For this review, take the finished solid that the model builds, in its own axes (mm). Face numbers are marked on the shaded views. A direction names the side the tool comes from. Coordinates: 2 decimals unless noted, no trailing zeros. Write each loop counter-clockwise with the first axis right and the second up, starting at its lowest first coordinate (ties: lowest second). Pieces come first, ordered by that corner, then holes. Notation, with made-up numbers: (30, 48.25) -> (47, 48.25) arc R21 ccw to (47, 58.25) -> close; hole circle Ø4 at (35, 5.25). An arc over 180 degrees is marked (long way). Put each result on its own line as item: value. Start each with the question number.
Item 1: To check wall thickness, follow L1, parallel to Z at x = 4.5, y = 6; L2, parallel to Z at x = 4.5, y = -18.5; L3, parallel to Z at x = -5, y = -5.5. State the ranges of each line that lie inside material, in increasing order.
Item 2: Insertion check: P1, Ø3, axis at x = 1.5, z = -46, coming from the -Y side; P2, Ø4, axis at x = 6, z = -1.5, coming from the +Y side; P3, Ø2, axis at y = 4, z = -17.5, coming from the -X side. Each pin has a flat end and moves straight along its axis. Give the tip position at first contact, or say it passes through.
Item 3: Consider section B-B on x = 2. Give the number of separate pieces and of enclosed holes in the cut face, and give its area (3 significant figures).
Item 4: For the marked faces 1, 2 and 3, list the 3-axis set-ups (+Z, -Z, +X, -X, +Y, -Y) from which the entire face can be reached by the end or side of a thin tool; tool diameter is ignored.
Item 5: Consider section A-A on z = 65. Give the boundary of the cut face in (x, y), and give its area (3 significant figures).
Item 6: The part is to be moulded in two halves that separate along Z. For the marked faces 4, 5 and 6, say which applies: +Z half, -Z half, draft (parallel to the pull), parting line (faces both ways), or undercut.
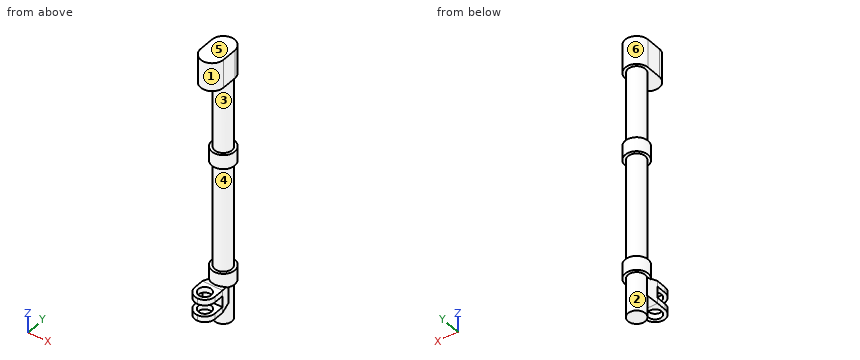
```python
from build123d import *

# Parameters (mm, degrees)
SKETCH1_R           = 6
BOSS_EXTRUDE1_DEPTH = 97.5
SKETCH4_W           = 14
SKETCH4_H           = 4
BOSS_EXTRUDE2_DEPTH = 14
SKETCH5_R           = 4.5
CUT_EXTRUDE1_DEPTH  = 4
CUT_EXTRUDE2_START  = -4
SKETCH6_R           = 4.5
CUT_EXTRUDE2_DEPTH  = 4
CUT_EXTRUDE3_START  = -16
CUT_EXTRUDE3_DEPTH  = 16
SKETCH8_R           = 8
BOSS_EXTRUDE3_DEPTH = 5
SKETCH9_R           = 8
SKETCH9_R_2         = 6
BOSS_EXTRUDE4_DEPTH = 20
BOSS_EXTRUDE5_START = 10
SKETCH11_R          = 8
BOSS_EXTRUDE5_DEPTH = 10


# Read off the part's stored shape, not the designer's step: Cut-Extrude3
with BuildPart() as part:
    # Sketch1 → Boss-Extrude1 (new, symmetric)
    with BuildSketch(Plane.XY):
        Circle(SKETCH1_R)
    extrude(amount=BOSS_EXTRUDE1_DEPTH, both=True)

    # Sketch2 → Loft1 section 0
    with BuildSketch(Plane(origin=(0, 0, 0), x_dir=(1, 0, 0), z_dir=(0, 1, 0))):
        with BuildLine():
            Line((-5, 82.5), (5, 82.5))
            Line((5, 82.5), (5, 70.5))
            Line((5, 70.5), (-5, 70.5))
            Line((-5, 70.5), (-5, 82.5))
        make_face()
    # Sketch3 → Loft1 section 1
    with BuildSketch(Plane(origin=(0, -10, 0), x_dir=(-1, 0, 0), z_dir=(0, 1, 0))):
        with BuildLine():
            Line((-7, -68.5), (7, -68.5))
            Line((7, -68.5), (7, -84.5))
            Line((7, -84.5), (-7, -84.5))
            Line((-7, -84.5), (-7, -68.5))
        make_face()
    loft()

    # Sketch4 → Boss-Extrude2 (add)
    with BuildSketch(Plane.XZ.offset(10)):
        with Locations((0, -70.5)):
            Rectangle(SKETCH4_W, SKETCH4_H)
        with Locations((0, -82.5)):
            Rectangle(SKETCH4_W, SKETCH4_H)
    extrude(amount=BOSS_EXTRUDE2_DEPTH)

    # Sketch5 → Cut-Extrude1 (cut)
    with BuildSketch(Plane(origin=(0, 0, -72.5), x_dir=(-1, 0, 0), z_dir=(0, 0, -1))):
        with Locations((0, -17)):
            Circle(SKETCH5_R)
    extrude(amount=-CUT_EXTRUDE1_DEPTH, mode=Mode.SUBTRACT)

    # Sketch6 → Cut-Extrude2 (cut)
    with BuildSketch(Plane.XY.offset(-80.5).offset(CUT_EXTRUDE2_START)):
        with Locations(Location((0, -17, 0), (0, 0, 180))):
            Circle(SKETCH6_R)
    extrude(amount=CUT_EXTRUDE2_DEPTH, mode=Mode.SUBTRACT)

    # Cut-Extrude3 outline → Cut-Extrude3 (cut)
    with BuildSketch(Plane.XY.offset(-68.5).offset(CUT_EXTRUDE3_START)):
        with BuildLine():
            ThreePointArc((7, -17), (4.949747468, -21.949747468), (0, -24))
            Line((0, -24), (7, -24))
            Line((7, -24), (7, -17))
        make_face()
        with BuildLine():
            ThreePointArc((0, -24), (-4.949747468, -21.949747468), (-7, -17))
            Line((-7, -17), (-7, -24))
            Line((-7, -24), (0, -24))
        make_face()
    extrude(amount=CUT_EXTRUDE3_DEPTH, mode=Mode.SUBTRACT)

    # Sketch8 → Boss-Extrude3 (add, symmetric)
    with BuildSketch(Plane.XY.offset(-65)):
        with Locations(Location((0, 0, 0), (0, 0, 220.893267512))):
            Circle(SKETCH8_R)
    extrude(amount=BOSS_EXTRUDE3_DEPTH, both=True)

    # Sketch9 → Boss-Extrude4 (add)
    # profile 1 of 2: a face of its own
    with BuildSketch(Plane.XY.offset(97.5)):
        with Locations(Location((0, 0, 0), (0, 0, 220.893267512))):
            Circle(SKETCH9_R)
        Circle(SKETCH9_R_2, mode=Mode.SUBTRACT)
    # profile 2 of 2: a face of its own
    with BuildSketch(Plane.XY.offset(97.5)):
        with BuildLine():
            ThreePointArc((8, 0), (0, -8), (-8, 0))
            Line((-8, 0), (-8, -10.315788333))
            ThreePointArc((-8, -10.315788333), (0, -18.315788333), (8, -10.315788333))
            Line((8, -10.315788333), (8, 0))
        make_face()
    extrude(amount=-BOSS_EXTRUDE4_DEPTH)

    # Sketch11 → Boss-Extrude5 (add)
    with BuildSketch(Plane.XY.offset(15).offset(BOSS_EXTRUDE5_START)):
        with Locations(Location((0, 0, 0), (0, 0, 220.893267512))):
            Circle(SKETCH11_R)
    extrude(amount=-BOSS_EXTRUDE5_DEPTH)


solid = part.part
```
Return value:
1. L1: -70 to -60, 15 to 25, 77.5 to 97.5
1. L2: -84.5 to -80.5, -72.5 to -68.5
1. L3: -83.6 to -60, 15 to 25, 77.5 to 97.5
2. P1: y = -6
2. P2: y = 4.47
2. P3: x = -5.2
3. separate pieces: 3
3. enclosed holes: 0
3. area: 2,690 mm^2
4. face 1: +Z, -Y
4. face 2: -Z
4. face 3: none
5. outline: circle Ø12 at (0, 0)
5. area: 113 mm^2
6. face 4: undercut
6. face 5: +Z half
6. face 6: draft
